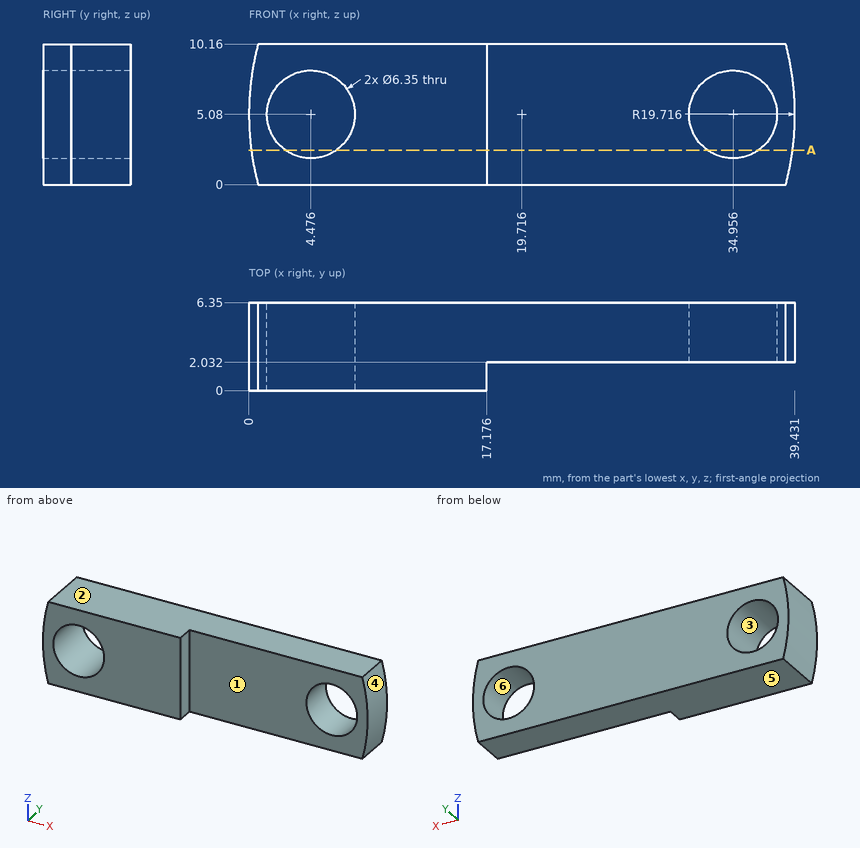
Answer from the drawing. Dimensions are ordinates in mm from the lowest x, y and z of the part. A direction names the side the tool comes from. Coordinates: 2 decimals unless noted, no trailing zeros.
1) For the marked faces 1 and 2, determine the directions among +Z, -Z, +X, -X, +Y, -Y from which every point of the face is accessible in a straight line to the end or side of a thin tool.
Results:
face 1: +Z, -Z, +X, -Y
face 2: +Z, +X, -X, +Y, -Y
2) Section A-A (z = 2.5) is taken. Give the number of separate pieces and of enclosed holes in the cut face, plus the area to 3 significant figures.
Results:
separate pieces: 3
enclosed holes: 0
area: 164 mm2
3) Flat-ended cylindrical pins translate along their axes: pin 1 (1 mm diameter, centred on y = 1, z = 3.5, fed in from +X); pin 2 (3 mm diameter, centred on x = 34, z = 7, fed in from -Y). Find the tip coordinate at first contact, or state that the pin passes through.
Results:
pin 1: stops at x = 17.18
pin 2: stops at y = 2.03
4) For a pull along Z with two mould halves and no side action, classify the marked faces 3, 4, 5 and 6 as +Z half, -Z half, draft (parallel to the pull), parting line (faces both ways), or undercut.
Results:
face 3: undercut
face 4: parting line
face 5: -Z half
face 6: undercut
5) Consider probe 1 along X at (y, z) = (4.5, 2.5) (1 decimal); probe 2 along X at (y, z) = (2.25, 4); probe 3 along Z at (x, y) = (33.5, 4.5). Determine where each line is inside the solid, lowest interval first.
Results:
probe 1: x = 0.2 to 2.6, 6.3 to 33.1, 36.8 to 39.3
probe 2: x = 0.03 to 1.49, 7.46 to 31.97, 37.94 to 39.4
probe 3: z = 0 to 2.26, 7.9 to 10.16
